from build123d import *

# Parameters (mm, degrees)
EXTRUDE009_DEPTH = 4
SKETCH002_R      = 8.31
SKETCH002_R_2    = 6.23
EXTRUDE002_DEPTH = 2


with BuildPart() as obj1:
    # Sketch012 (on Face8 of Extrude002) → Extrude009 (new body)
    with BuildSketch(Plane.XY.offset(2)):
        with BuildLine():
            ThreePointArc((26.8733973411, -32.9252261245), (35.4651440174, -23.4195123738), (40.8333333333, -11.7851130198))
            ThreePointArc((40.8333333333, -11.7851130198), (47.7113101314, -18.8477611751), (56.9484135086, -22.2921021863))
            Line((56.9484135086, -22.2921021863), (26.8733973411, -32.9252261245))
        make_face()
        with BuildLine():
            ThreePointArc((56.9484135086, 22.2921021863), (47.7113101314, 18.8477611751), (40.8333333333, 11.7851130198))
            ThreePointArc((40.8333333333, 11.7851130198), (35.4651440174, 23.4195123738), (26.8733973411, 32.9252261245))
            Line((56.9484135086, 22.2921021863), (26.8733973411, 32.9252261245))
        make_face()
    extrude(amount=EXTRUDE009_DEPTH)


with BuildPart() as base001:
    # Sketch002 → Extrude002 (new body)
    with BuildSketch(Plane.XY):
        with BuildLine():
            ThreePointArc((13.3333333333, 37.7123616633), (-40, 0), (13.3333333333, -37.7123616633))
            Line((66.6666666667, -18.8561808316), (13.3333333333, -37.7123616633))
            ThreePointArc((66.6666666667, -18.8561808316), (80, 0), (66.6666666667, 18.8561808316))
            Line((13.3333333333, 37.7123616633), (66.6666666667, 18.8561808316))
        make_face()
        Circle(SKETCH002_R, mode=Mode.SUBTRACT)
        with Locations((60, 0)):
            Circle(SKETCH002_R_2, mode=Mode.SUBTRACT)
    extrude(amount=EXTRUDE002_DEPTH)

    # Fusion002: union obj1
    add(obj1.part)


solid = base001.part
The listing builds one solid part. Answer for the finished solid, in the listing's coordinates (mm). A direction names the side the tool comes from. Give positions to 0.01 mm unless a question says otherwise; leave off trailing zeros. Order: outer loops, then holes, each group sorted by start corner. A loop starts at its lowest first (then second) coordinate and runs counter-clockwise, first axis right, second up. Notation, with made-up numbers: (58, 31) - (78, 31) arc R12 ccw to (78, 37) - close; hole circle Ø1 at (-5, 44.5). An arc over 180 degrees is marked (long way). One line per item, written item: value. Start each with the question number.
1) A cutting plane is placed at D-D on y = -13.5. Give the vertices of the cut face in (x, z), then the cut area to 3 significant figures.
2) Given pin 1 Ø3 at (y, z) = (6.5, 2.5) entering from +X; pin 2 Ø14.5 at (x, y) = (60, 0) entering from +Z, each flat-ended and moving along its own axis, determine where each tip first touches the part or whether it passes through.
3) A cutting plane is placed at C-C on x = 0. Give the vertices of the cut face in (y, z).
4) Find the intervals of material crossed by L1, parallel to Y at x = 0, z = 1.05; L2, parallel to Z at x = 52.5, y = -2; L3, parallel to Y at x = 60, z = 0.6, in increasing order.
5) The mould has two halves that part along Y. Classify faces 4 (the face through (80, 0, 1)), 5 (the face through (53.776, 0.274, 0.986)), 6 (the face through (40.373, -28.152, 2.291)), 7 (the face through (42, 23, 6)): released by +Y, released by -Y, zero draft, split by the parting line, or undercut.
6) A cutting plane is placed at B-B on z = 5.1. Give the vertices of the cut face in (x, y), then the cut area to 3 significant figures.
7) A tool of negligible diameter and unlimited length cuts with its end or side. For faces 1 (the face through (7.926, 2.496, 0.986)), 2 (the face through (47.828, 18.923, 3.972)), 3 (the face through (35.366, -23.57, 3.972)), from which of +Z, -Z, +X, -X, +Y, -Y can it reach the whole face along a straight path? Write none if from no direction.
8) A cutting plane is placed at A-A on y = 0. Give the vertices of the cut face in (x, z).
Answer sheet:
1. outline: (-37.65, 0) - (74.76, 0) - (74.76, 2) - (42, 2) - (42, 6) - (40.3, 6) - (40.3, 2) - (-37.65, 2) - close
1. area: 232 mm2
2. pin 1: stops at x = 79.34
2. pin 2: stops at z = 2
3. outline: (-40, 0) - (-8.31, 0) - (-8.31, 2) - (-40, 2) - close; (8.31, 0) - (40, 0) - (40, 2) - (8.31, 2) - close
4. L1: y = -40 to -8.31, 8.31 to 40
4. L2: z = 0 to 2
4. L3: y = -21.21 to -6.23, 6.23 to 21.21
5. face 4: split by the parting line
5. face 5: undercut
5. face 6: released by -Y
5. face 7: zero draft
6. outline: (26.87, -32.93) - (56.95, -22.29) arc R22.5 cw to (40.83, -11.79) arc R42.5 cw to start; (26.87, 32.93) arc R42.5 cw to (40.83, 11.79) arc R22.5 cw to (56.95, 22.29) - close
6. area: 366 mm2
7. face 1: +Z, -Z
7. face 2: +Z, +X
7. face 3: +Z, -X
8. outline: (-40, 0) - (-8.31, 0) - (-8.31, 2) - (-40, 2) - close; (8.31, 0) - (53.77, 0) - (53.77, 2) - (8.31, 2) - close; (66.23, 0) - (80, 0) - (80, 2) - (66.23, 2) - close
